Geometry check sheet. Reference: the model listing, model coordinates, mm. Face numbers are marked on the shaded views. A direction names the side the tool comes from. Round coordinates to 2 decimals unless told otherwise and drop trailing zeros. Order: outer loops, then holes, each group sorted by start corner. A loop starts at its lowest first (then second) coordinate and runs counter-clockwise, first axis right, second up.
(1) Go/stop test with flat-tipped pins: pin 1 (1.2 mm diameter, centred on x = 0.5, y = -20.5, fed in from +Z); pin 2 (1.5 mm diameter, centred on x = 4.5, y = -19, fed in from +Z); pin 3 (4.5 mm diameter, centred on x = 0, y = 20, fed in from -Z); pin 4 (1.2 mm diameter, centred on x = 0, y = 19, fed in from +Z). Record where each tip stops, or that it passes through.
(2) Material ranges on line 1 along Y through (x, z) = (0, 0.65); line 2 along X through (y, z) = (20, 1.7); line 3 along X through (y, z) = (-6.5, 6.5), recorded low to high.
(3) Set-up check for the marked faces 5 and 6: record each of +Z, -Z, +X, -X, +Y, -Y from which the full face is reachable in a straight line by a thin tool's end or side.
(4) Release check for a two-part mould opening along X. For the marked faces 1, 2, 3 and 4 record: +X half, -X half, draft (parallel to the pull), parting line (faces both ways), or undercut.
(5) Sectioned sample at D-D (z = 5). Give the number of separate pieces and of enclosed holes in the cut face, plus the area to 3 significant figures.
(6) Sectioned sample at C-C (y = 2). Record the boundary of the cut face in (x, z), plus the area to 3 significant figures.
(7) Sectioned sample at B-B (y = 20). Record the boundary of the cut face in (x, z).
Autodesk Inventor part; units mm, degrees
ref_plane "Arbeitsebene1" through (-6, 25, 0) normal (0.4226, 0, 0.9063) x (0.9063, 0, -0.4226)
ref_plane "YZ Plane" through (0, 0, 0) normal (1, 0, 0) x (0, 1, 0)
ref_plane "XZ Plane" through (0, 0, 0) normal (0, 1, 0) x (-1, 0, 0)
sketch "Skizze1" plane through (0, 0, 0) normal (0, 0, 1) x (1, 0, 0)
  line L0 (-6, -25) -> (6, -25)
  line L1 (6, -25) -> (6, 25)
  line L2 (6, 25) -> (-6, 25)
  line L3 (-6, 25) -> (-6, -25)
  line L4 (-6, -25) -> (6, 25) construction
  line L5 (6, -25) -> (-6, 25) construction
  line L6 (0, 20) -> (0, -20)
  point P0 (0, 0)
  point P1 (0, 0)
  dimension "d0" = 40
  dimension "d1" = 12
  dimension "d2" = 50
extrude "Extrusion1" add sketch "Skizze1" along normal blind 10
sketch "Skizze3" plane through (0, 0, 10) normal (0, 0, 1) x (1, 0, 0)
  line L0 (-6, -25) -> (6, -25)
  line L1 (6, -25) -> (6, 25)
  line L2 (6, 25) -> (-6, 25)
  line L3 (-6, 25) -> (-6, -25)
  point P0 (0, 0)
  point P1 (0, -20)
  point P2 (0, 20)
sketch "Skizze2" plane through (-6, -25, 0) normal (0, -1, 0) x (1, 0, 0)
  line L0 (0, 0) -> (12, 0)
  line L1 (12, 0) -> (12, 10)
  line L2 (0, 10) -> (12, 10)
  line L3 (0, 0) -> (0, 10)
  line L4 (0, 10) -> (12, 4.4043)
  point P0 (6, 0)
  dimension "d5" = 25
extrude "Extrusion2" cut sketch "Skizze2" against normal through all contours L2 L1 L4
hole "Bohrung1" at (0, 20, 10) at (0, -20, 10) direction (0, 0, -1) diameter 3 end through all counterbore diameter 4 counterbore depth 7
sketch "Skizze4" plane through (-6, -25, 10) normal (0.4226, 0, 0.9063) x (0.9063, 0, -0.4226)
  ellipse E0 centre (6.6203, 45) end of major axis (8.827, 45) minor radius 2
  ellipse E1 centre (6.6203, 5) end of major axis (8.827, 5) minor radius 2
  line L0 (0, 50) -> (13.2405, 50)
  line L1 (0, 50) -> (0, 0)
  line L2 (13.2405, 0) -> (0, 0)
  line L3 (13.2405, 50) -> (13.2405, 0)
  line L4 (6.6203, 12.5) -> (6.6203, 37.5)
  line L5 (0, 50) -> (0, 0)
  line L6 (0, 25) -> (13.2405, 25)
  line L7 (13.2405, 50) -> (13.2405, 0)
  point P0 (9.664, 25)
  point P1 (6.6203, 25)
  dimension "d15" = 25
hole "Bohrung2" at (0, -12.5, 7.2022) at (0, 12.5, 7.2022) direction (-0.4226, 0, -0.9063) diameter 3 end through all
ref_plane "Arbeitsebene1" through (-6, 25, 0) normal (0.4226, 0, 0.9063) x (0.9063, 0, -0.4226)
sketch "Skizze5" plane through (-6, 25, 0) normal (0.4226, 0, 0.9063) x (0.9063, 0, -0.4226)
  circle A0 centre (2.3941, -37.5) radius 1.5
  circle A1 centre (2.3941, -12.5) radius 1.5
  ellipse E0 centre (2.3941, -5) end of major axis (4.6008, -5) minor radius 2
  ellipse E1 centre (2.3941, -45) end of major axis (4.6008, -45) minor radius 2
  line L0 (-4.2262, 0) -> (9.0144, 0)
  line L1 (-4.2262, 0) -> (-4.2262, -50)
  line L2 (9.0144, -50) -> (-4.2262, -50)
  line L3 (9.0144, 0) -> (9.0144, -50)
  point P0 (5.4378, -25)
hole "Bohrung3" at (-3.8302, 12.5, -1.0118) at (-3.8302, -12.5, -1.0118) direction (0.4226, 0, 0.9063) diameter 3 end through all counterbore diameter 4 counterbore depth 5
properties part number "Mount"
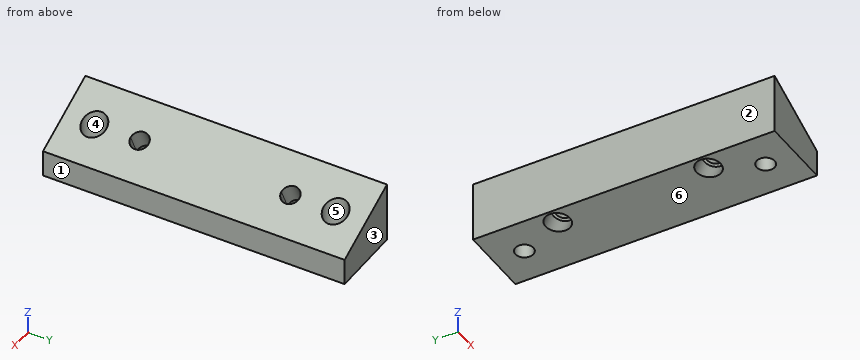
Answer below:
1. pin 1: passes through
1. pin 2: stops at z = 5.45
1. pin 3: stops at z = 0
1. pin 4: stops at z = 3
2. line 1: y = -25 to -21.5, -18.5 to 18.5, 21.5 to 25
2. line 2: x = -6 to -1.5, 1.5 to 6
2. line 3: x = -6 to 1.51
3. face 5: +Z
3. face 6: -Z, +X, -X, +Y, -Y
4. face 1: +X half
4. face 2: -X half
4. face 3: draft
4. face 4: undercut
5. separate pieces: 1
5. enclosed holes: 4
5. area: 495 mm2
6. outline: (-6, 0) - (6, 0) - (6, 4.4) - (-6, 10) - close
6. area: 86.4 mm2
7. outline: (-6, 0) - (-1.5, 0) - (-1.5, 3) - (-2, 3) - (-2, 8.13) - (-6, 10) - close; (1.5, 0) - (6, 0) - (6, 4.4) - (2, 6.27) - (2, 3) - (1.5, 3) - close
